Input: part model. Units: mm. Frame: model coordinates. A direction names the side the tool comes from. Round coordinates to 2 decimals unless told otherwise and drop trailing zeros. Order: outer loops, then holes, each group sorted by start corner. A loop starts at its lowest first (then second) coordinate and runs counter-clockwise, first axis right, second up. Notation, with made-up numbers: (24, 7.25) -> (51, 7.25) arc R26 cw to (51, 21.25) -> close; hole circle Ø8 at (25.5, 78). An arc over 180 degrees is marked (long way). Use a Markdown table: item, result.
from build123d import *

# Parameters (mm, degrees)
F0_R     = 34.4760551883
F1_DEPTH = 25.4
F1_TAPER = 40
F2_R     = 15.4170929596
F3_DEPTH = 217.2726094723


with BuildPart() as f1:
    # F0 (on Top) → F1 (new body)
    with BuildSketch(Plane.XY):
        Circle(F0_R)
    extrude(amount=F1_DEPTH, taper=F1_TAPER)

    # F2 (on Top) → F3 (join)
    with BuildSketch(Plane.XY):
        Circle(F2_R)
    extrude(amount=F3_DEPTH)

    # F4 (on Right) → F5 (revolve, cut)
    with BuildSketch(Plane.YZ):
        Polygon((9.2559680343, 224.6120274067), (7.9776421189, 217.2289937735), (15.5677124858, 207.9138755798), (24.6758013964, 207.9138755798), (24.6758013964, 224.6120274067), align=None)
    revolve(axis=Axis((0, 0, 227.7240306139), (0, 0, 1)), mode=Mode.SUBTRACT)


solid = f1.part
1) Cut plane A-A on y = 0. Return loops of the section in (x, z), and give its area (3 significant figures).
Answer key:
| item | result |
|---|---|
| outline | (-34.48, 0) -> (34.48, 0) -> (15.42, 22.71) -> (15.42, 208.1) -> (7.98, 217.23) -> (7.99, 217.27) -> (-7.99, 217.27) -> (-7.98, 217.23) -> (-15.42, 208.1) -> (-15.42, 22.71) -> close |
| area | 7,060 mm^2 |
2) Contact query for flat-ended pins moving along their axis: P1, Ø4, axis at x = 23, y = -8, coming from the +Z side; P2, Ø1.5, axis at x = 0, z = 101, coming from the +Y side; P3, Ø1.5, axis at x = 18, y = -14, coming from the +Z side. Output: stop coordinate, or through.
Answer key:
| item | result |
|---|---|
| P1 | stops at z = 14.45 |
| P2 | stops at y = 15.42 |
| P3 | stops at z = 14.8 |
3) Set-up query: faces 1 (the face through (0, 0, 0)), 2 (the face through (14.705, 4.631, 114.108)). Return all of +Z, -Z, +X, -X, +Y, -Y with unobstructed straight access to the full face (end or side cutting, diameter ignored); none if empty.
Answer key:
| item | result |
|---|---|
| face 1 | -Z, +X, -X, +Y, -Y |
| face 2 | +Z |
4) Cut plane C-C on z = 196.5. Return loops of the section in (x, y).
Answer key:
| item | result |
|---|---|
| outline | circle Ø30.83 at (0, 0) |
5) Ray query, probe 1 along Z at (x, y) = (-14, 26); probe 2 along X at (y, z) = (-6.5, 72); probe 3 along X at (y, z) = (14, 188.5). Return the intervals inside material, ascending.
Answer key:
| item | result |
|---|---|
| probe 1 | z = 0 to 5.89 |
| probe 2 | x = -13.98 to 13.98 |
| probe 3 | x = -6.46 to 6.46 |
